Verification items for the finished model (mm, model axes). Coordinates: 2 decimals unless noted, no trailing zeros. Write item = value, one per line. Start each with the question number.
(1) Section check A-A (z = 21). State how many separate pieces and enclosed holes the cut face has, plus the area to 3 significant figures.
(2) Gauge pin test, flat end, axial feed: pin 1 Ø7.5 at (x, z) = (-6, 33) entering from +Y. Record the tip position at first contact, or that the pin passes through.
(3) Material ranges on probe 1 along X at (y, z) = (67.5, 25.5); probe 2 along X at (y, z) = (95.5, 4.5); probe 3 along Y at (x, z) = (-69.5, 10), recorded low to high. Write a range as [from, to].
```python
from build123d import *

# Parameters (mm, degrees)
ESQUISSE1_W             = 320
ESQUISSE1_H             = 200
BOSS_EXTRU_1_DEPTH      = 60
ESQUISSE3_R             = 2
ESQUISSE3_W             = 6
ESQUISSE3_H             = 12
ENL_V_MAT_EXTRU_2_DEPTH = 60
CHANFREIN1_SIZE         = 40
ESQUISSE6_R             = 1.5
ENL_V_MAT_EXTRU_3_DEPTH = 60


with BuildPart() as part:
    # Esquisse1 → Boss.-Extru.1 (new body)
    with BuildSketch(Plane.XY):
        with Locations((-160, 100)):
            Rectangle(ESQUISSE1_W, ESQUISSE1_H)
    extrude(amount=BOSS_EXTRU_1_DEPTH)

    # Esquisse3 → Enlèv. mat.-Extru.2 (cut)
    with BuildSketch(Plane(origin=(0, 0, 0), x_dir=(-1, 0, 0), z_dir=(0, 0, -1))):
        with Locations((70.1, 102)):
            Circle(ESQUISSE3_R)
        with Locations((91.24, 102)):
            Circle(ESQUISSE3_R)
        with Locations((118.24, 102)):
            Circle(ESQUISSE3_R)
        with Locations(Location((201.76, 102, 0), (0, 0, 180))):
            Circle(ESQUISSE3_R)
        with Locations(Location((228.76, 102, 0), (0, 0, 180))):
            Circle(ESQUISSE3_R)
        with Locations(Location((249.9, 102, 0), (0, 0, 180))):
            Circle(ESQUISSE3_R)
        with Locations((70.1, 88)):
            Rectangle(ESQUISSE3_W, ESQUISSE3_H)
        with Locations((70.1, 116)):
            Rectangle(ESQUISSE3_W, ESQUISSE3_H)
        with Locations((91.24, 88)):
            Rectangle(ESQUISSE3_W, ESQUISSE3_H)
        with Locations((91.24, 116)):
            Rectangle(ESQUISSE3_W, ESQUISSE3_H)
        with Locations((118.24, 88)):
            Rectangle(ESQUISSE3_W, ESQUISSE3_H)
        with Locations((118.24, 116)):
            Rectangle(ESQUISSE3_W, ESQUISSE3_H)
        with Locations((201.76, 88)):
            Rectangle(ESQUISSE3_W, ESQUISSE3_H)
        with Locations((201.76, 116)):
            Rectangle(ESQUISSE3_W, ESQUISSE3_H)
        with Locations((228.76, 88)):
            Rectangle(ESQUISSE3_W, ESQUISSE3_H)
        with Locations((228.76, 116)):
            Rectangle(ESQUISSE3_W, ESQUISSE3_H)
        with Locations((249.9, 88)):
            Rectangle(ESQUISSE3_W, ESQUISSE3_H)
        with Locations((249.9, 116)):
            Rectangle(ESQUISSE3_W, ESQUISSE3_H)
    extrude(amount=-ENL_V_MAT_EXTRU_2_DEPTH, mode=Mode.SUBTRACT)

    # Chanfrein1
    chanfrein1_edges = [part.edges().sort_by_distance(p)[0] for p in [
        (-320, 200, 30),
        (0, 200, 30),
    ]]
    chamfer(chanfrein1_edges, length=CHANFREIN1_SIZE)

    # Esquisse6 → Enlèv. mat.-Extru.3 (cut)
    with BuildSketch(Plane.XY.offset(60)):
        with Locations((-260.750206469, 189.977960498)):
            Circle(ESQUISSE6_R)
        with Locations((-210.375103235, 189.977960498)):
            Circle(ESQUISSE6_R)
        with Locations(Location((-109.624896765, 189.977960498, 0), (0, 0, 180))):
            Circle(ESQUISSE6_R)
        with Locations(Location((-59.249793531, 189.977960498, 0), (0, 0, 180))):
            Circle(ESQUISSE6_R)
        with Locations((-303, 47)):
            Circle(ESQUISSE6_R)
        with Locations((-293, 47)):
            Circle(ESQUISSE6_R)
        with Locations(Location((-293, 127.148940914, 0), (0, 0, 180))):
            Circle(ESQUISSE6_R)
        with Locations(Location((-303, 127.148940914, 0), (0, 0, 180))):
            Circle(ESQUISSE6_R)
        with Locations(Location((-27, 47, 0), (0, 0, 180))):
            Circle(ESQUISSE6_R)
        with Locations(Location((-17, 47, 0), (0, 0, 180))):
            Circle(ESQUISSE6_R)
        with Locations((-17, 127.148940914)):
            Circle(ESQUISSE6_R)
        with Locations((-27, 127.148940914)):
            Circle(ESQUISSE6_R)
        Polygon((-287, 120), (-309, 120), (-309, 110), (-316, 110), (-316, 64), (-309, 64), (-309, 54), (-287, 54), (-287, 36.405681604), (-282.9, 36.405681604), (-282.9, 94.405681604), (-287, 94.405681604), align=None)
        Polygon((-33, 36.405681604), (-33, 54), (-11, 54), (-11, 64), (-4, 64), (-4, 110), (-11, 110), (-11, 120), (-33, 120), (-33, 94.405681604), (-37.1, 94.405681604), (-37.1, 36.405681604), align=None)
    extrude(amount=-ENL_V_MAT_EXTRU_3_DEPTH, mode=Mode.SUBTRACT)


solid = part.part
```
Response:
q1.separate_pieces = 1
q1.enclosed_holes = 32
q1.area = 57,400 mm2
q2.pin_1 = 169.75
q3.probe_1 = [-320, -316], [-282.9, -37.1], [-4, 0]
q3.probe_2 = [-320, -316], [-287, -33], [-4, 0]
q3.probe_3 = [0, 82], [94, 100.09], [103.91, 110], [122, 200]
